Geometry: final body of the model. Coordinates: model frame, mm. Face numbers are marked on the shaded views. A direction names the side the tool comes from. Round coordinates to 2 decimals unless told otherwise and drop trailing zeros. Order: outer loops, then holes, each group sorted by start corner. A loop starts at its lowest first (then second) coordinate and runs counter-clockwise, first axis right, second up. Notation, with made-up numbers: M 85,3 L 133,3 A15 ccw 133,13 Z; hole C 16.25,-12 d10. An arc over 180 degrees is marked long. Put each result on its own line as item: value. Start each with the question number.
1) Draft query along Y for the marked faces 1, 2, 3 and 4. Return one class per face: pulls with the +Y half, pulls with the -Y half, needs draft (parallel to the pull), parting line crosses it, or undercut.
2) First-contact query: P1, Ø10, axis at y = 6.5, z = 1, coming from the -X side; P2, Ø4.5, axis at x = -8.585, z = 10.165, coming from the +Y side; P3, Ø10, axis at x = -62, z = 3.5, coming from the -Y side. Flat tips, straight axial feed; report the tip coordinate or a pass-through.
3) Access query for the marked faces 5, 6, 7, 8 and 9. Directions: +Z, -Z, +X, -X, +Y, -Y. A direction counts if a zero-diameter tool reaches every point of the face in a straight line with its end or side. Return the directions, or none.
4) Material intervals for probe 1 along X at (y, z) = (61.5, 14); probe 2 along Y at (x, z) = (-9.5, -0.5); probe 3 along X at (y, z) = (56.5, 16.5), sorted ascending. Write a range as [from, to].
5) Section D-D, the plane x = -33. Return loops of the section in (y, z).
6) Section B-B, the plane y = 25.5. Return loops of the section in (x, z) (3 decimals).
7) Section C-C, the plane y = 51.5. Return loops of the section in (x, z) (3 decimals), then the cut area to 3 significant figures.
8) Section A-A, the plane x = -14. Return loops of the section in (y, z) (3 decimals), then the cut area to 3 significant figures.
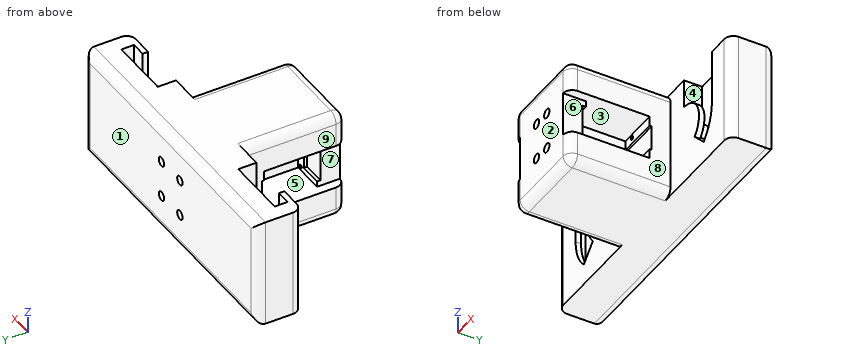
from build123d import *

# Parameters (mm, degrees)
BOSS_EXTRUDE1_DEPTH            = 30
BOSS_EXTRUDE1_DEPTH_BACK       = 30
CUT_REVOLVE2_START             = 59
CUT_REVOLVE2_DEPTH             = 7
CUT_REVOLVE2_START_2           = 56
CUT_REVOLVE2_2_DEPTH           = 3
CUT_EXTRUDE1_DEPTH             = 22.615
CUT_EXTRUDE2_REACH             = 130.69
CUT_EXTRUDE2_DIRECTION_2_DEPTH = 129.689548915
FILLET5_R                      = 5
FILLET6_R                      = 5
SKETCH7_W                      = 18.23
SKETCH7_H                      = 1.85
CUT_EXTRUDE3_DEPTH             = 17.32
SKETCH8_W                      = 20
SKETCH8_H                      = 24.63
CUT_EXTRUDE4_DEPTH             = 15.3
CUT_EXTRUDE5_REACH             = 119.733
SKETCH10_R                     = 1
SKETCH12_R                     = 2.5
CUT_EXTRUDE6_DEPTH             = 10.5
CUT_EXTRUDE7_REACH             = 119.733
SKETCH13_R                     = 1
SKETCH14_R                     = 2.5
CUT_EXTRUDE8_DEPTH             = 34.5


# Read off the part's stored shape, not the designer's step: Cut-Revolve2
with BuildPart() as part:
    # Sketch1 → Boss-Extrude1 (new, two sides: drawn at the far end of the back side and taken through both)
    with BuildSketch(Plane.XY.offset(-BOSS_EXTRUDE1_DEPTH_BACK)):
        Polygon((-25, 0), (-25, 56), (-80, 56), (-80, 81), (80, 81), (80, 56), (25, 56), (25, 0), align=None)
    extrude(amount=BOSS_EXTRUDE1_DEPTH + BOSS_EXTRUDE1_DEPTH_BACK)

    # Cut-Revolve2 outline → Cut-Revolve2 (cut)
    with BuildSketch(Plane(origin=(0, 0, 0), x_dir=(1, 0, 0), z_dir=(0, 1, 0)).offset(CUT_REVOLVE2_START)):
        with BuildLine():
            ThreePointArc((-37.5, -6), (-43.043277195, -2.296100594), (-41.742640687, 4.242640687))
            Line((-41.742640687, 4.242640687), (-61.54163056, 24.04163056))
            ThreePointArc((-61.54163056, 24.04163056), (-71.129711609, -5.004247907), (-53.5, -30))
            Line((-53.5, -30), (-37.5, -30))
            Line((-37.5, -30), (-37.5, -6))
        make_face()
    cut_revolve2 = extrude(amount=CUT_REVOLVE2_DEPTH, mode=Mode.SUBTRACT)

    # Cut-Revolve2 2 outline → Cut-Revolve2 2 (cut)
    with BuildSketch(Plane(origin=(0, 0, 0), x_dir=(1, 0, 0), z_dir=(0, 1, 0)).offset(CUT_REVOLVE2_START_2)):
        with BuildLine():
            Line((-37.5, -26), (-37.5, -14))
            ThreePointArc((-37.5, -14), (-50.434313455, -5.357568053), (-47.399494937, 9.899494937))
            Line((-47.399494937, 9.899494937), (-55.884776311, 18.384776311))
            ThreePointArc((-55.884776311, 18.384776311), (-61.520867845, -9.949769241), (-37.5, -26))
        make_face()
    cut_revolve2_2 = extrude(amount=CUT_REVOLVE2_2_DEPTH, mode=Mode.SUBTRACT)

    # Sketch4 → Cut-Extrude1 (cut)
    with BuildSketch(Plane.ZY.offset(25)):
        Polygon((12.315, 12.5), (-12.315, 12.5), (-12.315, 44.5), (-6.965, 44.5), (-6.965, 45.65), (7.015, 45.65), (7.015, 44.5), (12.315, 44.5), align=None)
    cut_extrude1 = extrude(amount=-CUT_EXTRUDE1_DEPTH, mode=Mode.SUBTRACT)

    # Mirror1: Cut-Extrude1 across plane
    add(cut_extrude1.mirror(Plane.ZY), mode=Mode.SUBTRACT)

    # Sketch5 → Cut-Extrude2 (cut, up to next)
    with BuildSketch(Plane.XY.offset(30), mode=Mode.PRIVATE) as cut_extrude2_sk1:
        Polygon((-63.5, 56), (-37.5, 56), (-37.5, 66), (-71.5, 66), (-71.5, 59), (-63.5, 59), align=None)
    cut_extrude2_tool1 = extrude(cut_extrude2_sk1.sketch, amount=-CUT_EXTRUDE2_REACH, mode=Mode.PRIVATE) & part.part
    cut_extrude2 = cut_extrude2_tool1.solids().sort_by_distance((-53.512658, 61.265823, 30))[0]
    add(cut_extrude2, mode=Mode.SUBTRACT)

    # Sketch5 → Cut-Extrude2 direction 2 (cut)
    with BuildSketch(Plane.XY.offset(30)):
        Polygon((-63.5, 56), (-37.5, 56), (-37.5, 66), (-71.5, 66), (-71.5, 59), (-63.5, 59), align=None)
    cut_extrude2_direction_2 = extrude(amount=CUT_EXTRUDE2_DIRECTION_2_DEPTH, mode=Mode.SUBTRACT)

    # Mirror4: Cut-Revolve2, Cut-Revolve2 2 across plane
    add(cut_revolve2.mirror(Plane.ZY), mode=Mode.SUBTRACT)
    add(cut_revolve2_2.mirror(Plane.ZY), mode=Mode.SUBTRACT)

    # Mirror2: Cut-Extrude2, Cut-Extrude2 direction 2 across plane
    add(cut_extrude2.mirror(Plane.ZY), mode=Mode.SUBTRACT)
    add(cut_extrude2_direction_2.mirror(Plane.ZY), mode=Mode.SUBTRACT)

    # Fillet5
    fillet5_edges = [part.edges().sort_by_distance(p)[0] for p in [
        (-80, 81, 0),
        (80, 81, 0),
        (0, 81, -30),
        (0, 81, 30),
    ]]
    fillet(fillet5_edges, radius=FILLET5_R)

    # Fillet6
    fillet6_edges = [part.edges().sort_by_distance(p)[0] for p in [
        (-25, 0, 0),
        (-80, 56, 0),
        (80, 56, 0),
        (25, 0, 0),
        (0, 0, 30),
        (25, 28, 30),
        (-25, 28, 30),
        (-25, 28, -30),
        (0, 0, -30),
        (25, 28, -30),
    ]]
    fillet(fillet6_edges, radius=FILLET6_R)

    # Sketch7 → Cut-Extrude3 (cut)
    with BuildSketch(Plane.ZY.offset(25)):
        with Locations((0, 11.575)):
            Rectangle(SKETCH7_W, SKETCH7_H)
    cut_extrude3 = extrude(amount=-CUT_EXTRUDE3_DEPTH, mode=Mode.SUBTRACT)

    # Mirror5: Cut-Extrude3 across plane
    add(cut_extrude3.mirror(Plane.ZY), mode=Mode.SUBTRACT)

    # Sketch8 → Cut-Extrude4 (cut)
    with BuildSketch(Plane.XZ):
        with Locations((-30, 0)):
            Rectangle(SKETCH8_W, SKETCH8_H)
        with Locations((30, 0)):
            Rectangle(SKETCH8_W, SKETCH8_H)
    extrude(amount=-CUT_EXTRUDE4_DEPTH, mode=Mode.SUBTRACT)

    # Sketch10 → Cut-Extrude5 (cut, up to next)
    with BuildSketch(Plane(origin=(0, 0, 0), x_dir=(-1, 0, 0), z_dir=(0, -1, 0)), mode=Mode.PRIVATE) as cut_extrude5_sk1:
        with Locations(Location((4.785, -10.165, 0), (0, 0, 90))):
            Circle(SKETCH10_R)
    cut_extrude5_tool1 = extrude(cut_extrude5_sk1.sketch, amount=-CUT_EXTRUDE5_REACH, mode=Mode.PRIVATE) & part.part
    # Sketch10 → Cut-Extrude5 (cut, up to next)
    with BuildSketch(Plane(origin=(0, 0, 0), x_dir=(-1, 0, 0), z_dir=(0, -1, 0)), mode=Mode.PRIVATE) as cut_extrude5_sk2:
        with Locations(Location((4.785, 10.165, 0), (0, 0, 180))):
            Circle(SKETCH10_R)
    cut_extrude5_tool2 = extrude(cut_extrude5_sk2.sketch, amount=-CUT_EXTRUDE5_REACH, mode=Mode.PRIVATE) & part.part
    # Sketch10 → Cut-Extrude5 (cut, up to next)
    with BuildSketch(Plane(origin=(0, 0, 0), x_dir=(-1, 0, 0), z_dir=(0, -1, 0)), mode=Mode.PRIVATE) as cut_extrude5_sk3:
        with Locations(Location((-4.785, 10.165, 0), (0, 0, 90))):
            Circle(SKETCH10_R)
    cut_extrude5_tool3 = extrude(cut_extrude5_sk3.sketch, amount=-CUT_EXTRUDE5_REACH, mode=Mode.PRIVATE) & part.part
    # Sketch10 → Cut-Extrude5 (cut, up to next)
    with BuildSketch(Plane(origin=(0, 0, 0), x_dir=(-1, 0, 0), z_dir=(0, -1, 0)), mode=Mode.PRIVATE) as cut_extrude5_sk4:
        with Locations((-4.785, -10.165)):
            Circle(SKETCH10_R)
    cut_extrude5_tool4 = extrude(cut_extrude5_sk4.sketch, amount=-CUT_EXTRUDE5_REACH, mode=Mode.PRIVATE) & part.part
    add(cut_extrude5_tool1.solids().sort_by_distance((-4.785, 0, 10.165))[0], mode=Mode.SUBTRACT)
    add(cut_extrude5_tool2.solids().sort_by_distance((-4.785, 0, -10.165))[0], mode=Mode.SUBTRACT)
    add(cut_extrude5_tool3.solids().sort_by_distance((4.785, 0, -10.165))[0], mode=Mode.SUBTRACT)
    add(cut_extrude5_tool4.solids().sort_by_distance((4.785, 0, 10.165))[0], mode=Mode.SUBTRACT)

    # Sketch12 → Cut-Extrude6 (cut)
    with BuildSketch(Plane.XZ):
        with Locations(Location((-4.785, 10.165, 0), (0, 0, 270))):
            Circle(SKETCH12_R)
        with Locations((-4.785, -10.165)):
            Circle(SKETCH12_R)
        with Locations(Location((4.785, -10.165, 0), (0, 0, 270))):
            Circle(SKETCH12_R)
        with Locations((4.785, 10.165)):
            Circle(SKETCH12_R)
    extrude(amount=-CUT_EXTRUDE6_DEPTH, mode=Mode.SUBTRACT)

    # Sketch13 → Cut-Extrude7 (cut, up to next)
    with BuildSketch(Plane(origin=(0, 81, 0), x_dir=(1, 0, 0), z_dir=(0, 1, 0)), mode=Mode.PRIVATE) as cut_extrude7_sk1:
        with Locations(Location((-8.585, 10.165, 0), (0, 0, 270))):
            Circle(SKETCH13_R)
    cut_extrude7_tool1 = extrude(cut_extrude7_sk1.sketch, amount=-CUT_EXTRUDE7_REACH, mode=Mode.PRIVATE) & part.part
    # Sketch13 → Cut-Extrude7 (cut, up to next)
    with BuildSketch(Plane(origin=(0, 81, 0), x_dir=(1, 0, 0), z_dir=(0, 1, 0)), mode=Mode.PRIVATE) as cut_extrude7_sk2:
        with Locations(Location((-8.585, -10.165, 0), (0, 0, 180))):
            Circle(SKETCH13_R)
    cut_extrude7_tool2 = extrude(cut_extrude7_sk2.sketch, amount=-CUT_EXTRUDE7_REACH, mode=Mode.PRIVATE) & part.part
    # Sketch13 → Cut-Extrude7 (cut, up to next)
    with BuildSketch(Plane(origin=(0, 81, 0), x_dir=(1, 0, 0), z_dir=(0, 1, 0)), mode=Mode.PRIVATE) as cut_extrude7_sk3:
        with Locations(Location((8.585, -10.165, 0), (0, 0, 270))):
            Circle(SKETCH13_R)
    cut_extrude7_tool3 = extrude(cut_extrude7_sk3.sketch, amount=-CUT_EXTRUDE7_REACH, mode=Mode.PRIVATE) & part.part
    # Sketch13 → Cut-Extrude7 (cut, up to next)
    with BuildSketch(Plane(origin=(0, 81, 0), x_dir=(1, 0, 0), z_dir=(0, 1, 0)), mode=Mode.PRIVATE) as cut_extrude7_sk4:
        with Locations((8.585, 10.165)):
            Circle(SKETCH13_R)
    cut_extrude7_tool4 = extrude(cut_extrude7_sk4.sketch, amount=-CUT_EXTRUDE7_REACH, mode=Mode.PRIVATE) & part.part
    add(cut_extrude7_tool1.solids().sort_by_distance((-8.585, 81, -10.165))[0], mode=Mode.SUBTRACT)
    add(cut_extrude7_tool2.solids().sort_by_distance((-8.585, 81, 10.165))[0], mode=Mode.SUBTRACT)
    add(cut_extrude7_tool3.solids().sort_by_distance((8.585, 81, 10.165))[0], mode=Mode.SUBTRACT)
    add(cut_extrude7_tool4.solids().sort_by_distance((8.585, 81, -10.165))[0], mode=Mode.SUBTRACT)

    # Sketch14 → Cut-Extrude8 (cut)
    with BuildSketch(Plane(origin=(0, 81, 0), x_dir=(1, 0, 0), z_dir=(0, 1, 0))):
        with Locations(Location((-8.585, 10.165, 0), (0, 0, 270))):
            Circle(SKETCH14_R)
        with Locations(Location((-8.585, -10.165, 0), (0, 0, 180))):
            Circle(SKETCH14_R)
        with Locations(Location((8.585, -10.165, 0), (0, 0, 270))):
            Circle(SKETCH14_R)
        with Locations(Location((8.585, 10.165, 0), (0, 0, 180))):
            Circle(SKETCH14_R)
    extrude(amount=-CUT_EXTRUDE8_DEPTH, mode=Mode.SUBTRACT)


solid = part.part
Result sheet:
1. face 1: pulls with the +Y half
1. face 2: pulls with the -Y half
1. face 3: undercut
1. face 4: undercut
2. P1: stops at x = -20
2. P2: stops at y = 46.5
2. P3: stops at y = 56
3. face 5: -X
3. face 6: +X, -Y
3. face 7: -X, -Y
3. face 8: +Z, -Z, +X, -Y
3. face 9: +Z, -Z, -X, -Y
4. probe 1: x = [-80, -71.5], [-37.5, 37.5], [71.5, 80]
4. probe 2: y = [0, 10.65], [45.65, 81]
4. probe 3: x = [-77.18, -63.5], [-37.5, 37.5], [63.5, 77.18]
5. outline: M 56,-30 L 76,-30 A5 ccw 81,-25 L 81,25 A5 ccw 76,30 L 56,30 Z
6. outline: M -25,-25 A5 ccw -20,-30 L 20,-30 A5 ccw 25,-25 L 25,-12.315 L 2.385,-12.315 L 2.385,12.315 L 25,12.315 L 25,25 A5 ccw 20,30 L -20,30 A5 ccw -25,25 L -25,12.315 L -2.385,12.315 L -2.385,-12.315 L -25,-12.315 Z
7. outline: M -25,-25 A5 ccw -20,-30 L 20,-30 A5 ccw 25,-25 L 25,25 A5 ccw 20,30 L -20,30 A5 ccw -25,25 Z; hole C -8.585,-10.165 d5; hole C -8.585,10.165 d5; hole C 8.585,-10.165 d5; hole C 8.585,10.165 d5
7. area: 2,900 mm2
8. outline: M 0,-25 A5 ccw 5,-30 L 76,-30 A5 ccw 81,-25 L 81,25 A5 ccw 76,30 L 5,30 A5 ccw 0,25 Z; hole M 10.65,-9.115 L 12.5,-9.115 L 12.5,-12.315 L 44.5,-12.315 L 44.5,-6.965 L 45.65,-6.965 L 45.65,7.015 L 44.5,7.015 L 44.5,12.315 L 12.5,12.315 L 12.5,9.115 L 10.65,9.115 Z
8. area: 4,000 mm2
